Work out the finished part from the listing and answer in its coordinate system (mm). A direction names the side the tool comes from. Give positions to 0.01 mm unless a question says otherwise; leave off trailing zeros. Loops run counter-clockwise (first coordinate to the right, second up) from the corner with the lowest first, then second, coordinate; pieces in that order, holes last.
from build123d import *

# Parameters (mm, degrees)
F0_W     = 44.45
F0_H     = 6.35
F0_W_2   = 6.35
F0_H_2   = 44.45
F1_DEPTH = 25.4
F2_R     = 4.960938
F3_DEPTH = 25.4
F5_R     = 3.2639
F6_DEPTH = 25.4


with BuildPart() as f1:
    # F0 (on Right) → F1 (new body)
    with BuildSketch(Plane.YZ):
        with Locations((-28.575, 3.175)):
            Rectangle(F0_W, F0_H)
        with Locations((-3.175, 3.175)):
            Rectangle(F0_W_2, F0_H)
        with Locations((-3.175, 28.575)):
            Rectangle(F0_W_2, F0_H_2)
    extrude(amount=F1_DEPTH)

    # F2 (on face) → F3 (cut)
    with BuildSketch(Plane.XY.offset(6.35)):
        with Locations((12.7, -33.3375)):
            Circle(F2_R)
    extrude(amount=-F3_DEPTH, mode=Mode.SUBTRACT)

    # F5 (on face) → F6 (cut)
    with BuildSketch(Plane.XZ.offset(6.35)):
        with Locations((12.7, 12.7)):
            Circle(F5_R)
        with Locations((12.7, 38.1)):
            Circle(F5_R)
    extrude(amount=-F6_DEPTH, mode=Mode.SUBTRACT)


solid = f1.part
Item 1: Find section D-D, the plane z = 19.5. Write down the section's boundary in (x, y).
Item 2: Find section C-C, the plane y = -32. Write down the section's boundary in (x, z).
Item 3: Find section A-A, the plane x = 12.7. Write down the section's boundary in (y, z), plus the area to 3 significant figures.
Item 4: Find section B-B, the plane z = 38.1. Write down the section's boundary in (x, y).
Item 5: Flat-ended cylindrical pins translate along their axes: pin 1 Ø5 at (x, y) = (19, -43) entering from +Z; pin 2 Ø6 at (x, z) = (12.7, 38.1) entering from +Y. Find the tip coordinate at first contact, or state that the pin passes through.
Item 6: For faces 4 (the face through (13, -50.8, 3)), 5 (the face through (13, -6.35, 28)), determine the directions among +Z, -Z, +X, -X, +Y, -Y from which every point of the face is accessible in a straight line to the end or side of a thin tool.
Item 7: Consider line 1 (Z direction, x = 12.7, y = -3.5); line 2 (Y direction, x = 12.7, z = 2.5); line 3 (X direction, y = -2, z = 38). Determine where each line is inside the solid, lowest interval first.
Item 8: Determine the mould class of faces 1 (the face through (25.4, -14, 5)), 2 (the face through (10.11, -3.219, 10.714)), 3 (the face through (13, -26, 0)) for opening direction Z: released by +Z, released by -Z, zero draft, split by the parting line, or undercut.
Ans:
1. outline: (0, -6.35) - (25.4, -6.35) - (25.4, 0) - (0, 0) - close
2. outline: (0, 0) - (7.92, 0) - (7.92, 6.35) - (0, 6.35) - close; (17.48, 0) - (25.4, 0) - (25.4, 6.35) - (17.48, 6.35) - close
3. outline: (-50.8, 0) - (-38.3, 0) - (-38.3, 6.35) - (-50.8, 6.35) - close; (-28.38, 0) - (0, 0) - (0, 9.44) - (-6.35, 9.44) - (-6.35, 6.35) - (-28.38, 6.35) - close; (-6.35, 15.96) - (0, 15.96) - (0, 34.84) - (-6.35, 34.84) - close; (-6.35, 41.36) - (0, 41.36) - (0, 50.8) - (-6.35, 50.8) - close
3. area: 459 mm2
4. outline: (0, -6.35) - (9.44, -6.35) - (9.44, 0) - (0, 0) - close; (15.96, -6.35) - (25.4, -6.35) - (25.4, 0) - (15.96, 0) - close
5. pin 1: stops at z = 6.35
5. pin 2: passes through
6. face 4: +Z, -Z, +X, -X, -Y
6. face 5: +Z, +X, -X, -Y
7. line 1: z = 0 to 9.44, 15.96 to 34.84, 41.36 to 50.8
7. line 2: y = -50.8 to -38.3, -28.38 to 0
7. line 3: x = 0 to 9.44, 15.96 to 25.4
8. face 1: zero draft
8. face 2: undercut
8. face 3: released by -Z
